Verification items for the finished model (mm, model axes). A direction names the side the tool comes from. Round coordinates to 2 decimals unless told otherwise and drop trailing zeros. Order: outer loops, then holes, each group sorted by start corner. A loop starts at its lowest first (then second) coordinate and runs counter-clockwise, first axis right, second up. Notation, with made-up numbers: M 73,-3.5 L 97,-3.5 A12 cw 97,2.5 Z; hole C 81,48 d11. An arc over 180 degrees is marked long. Return JSON: item names as keys, results as strings. Group by question number.
from build123d import *

# Parameters (mm, degrees)
SKETCH1_W           = 40
SKETCH1_H           = 20
BOSS_EXTRUDE1_DEPTH = 3
FILLET1_R           = 15


with BuildPart() as part:
    # Sketch1 → Boss-Extrude1 (new body)
    with BuildSketch(Plane.XY):
        Polygon((52, 50.85), (52, 47.85), (58, 47.85), (58, 50.85), (110, 50.85), (110, 0), (58, 0), (58, 3), (52, 3), (52, 0), (0, 0), (0, 50.85), align=None)
        with Locations((55, 25.425)):
            Rectangle(SKETCH1_W, SKETCH1_H, mode=Mode.SUBTRACT)
    extrude(amount=BOSS_EXTRUDE1_DEPTH)

    # Fillet1
    fillet1_edges = [part.edges().sort_by_distance(p)[0] for p in [
        (0, 0, 1.5),
        (110, 0, 1.5),
        (110, 50.85, 1.5),
        (0, 50.85, 1.5),
    ]]
    fillet(fillet1_edges, radius=FILLET1_R)


solid = part.part
1. Cross-section at D-D (y = 10). Enter the section's corners in (x, z), plus the area to 3 significant figures.
2. Access from +Z, -Z, +X, -X, +Y, -Y to the whole of each face (thin tool, end or side, straight path). Record for faces 4 (the face through (52, 2, 1)), 5 (the face through (52, 49, 1)), 6 (the face through (75, 25, 1)), 7 (the face through (33, 50.85, 1)).
3. Thickness scan on line 1 along Y through (x, z) = (50.5, 2.3) (3 decimals); line 2 along Y through (x, z) = (55, 0.75) (3 decimals); line 3 along X through (y, z) = (32, 2.8). Record the ranges inside material, lowest first. Write a range as from..to.
4. Go/stop test with flat-tipped pins: pin 1 (1.5 mm diameter, centred on x = 54, z = 2, fed in from -Y); pin 2 (0.9 mm diameter, centred on y = 1.5, z = 1, fed in from -X). Record where each tip stops, or that it passes through.
5. Draft check along X on faces 1 (the face through (34, 0, 1)), 2 (the face through (58, 1, 1)), 3 (the face through (4.28, 4.51, 1.52)). Enter one of: +X half, -X half, draft (parallel to the pull), parting line (faces both ways), or undercut.
6. Cross-section at C-C (y = 19). Enter the section's corners in (x, z).
7. Cross-section at B-B (z = 2.2). Enter the section's corners in (x, y) (3 decimals), plus the area to 3 significant figures.
8. Cross-section at A-A (x = 46.5). Enter the section's corners in (y, z) (3 decimals).
Computed:
{
 "1": {"outline": "M 0.86,0 L 109.14,0 L 109.14,3 L 0.86,3 Z", "area": "325 mm²"},
 "2": {"face 4": "+Z, -Z, -Y", "face 5": "+Z, -Z, +Y", "face 6": "+Z, -Z", "face 7": "+Z, -Z, +X, -X, +Y"},
 "3": {"line 1": "y = 0..15.425, 35.425..50.85", "line 2": "y = 3..15.425, 35.425..47.85", "line 3": "x = 0..35, 75..110"},
 "4": {"pin 1": "stops at y = 3", "pin 2": "stops at x = 7.6"},
 "5": {"face 1": "draft", "face 2": "undercut", "face 3": "-X half"},
 "6": {"outline": "M 0,0 L 35,0 L 35,3 L 0,3 Z; M 75,0 L 110,0 L 110,3 L 75,3 Z"},
 "7": {"outline": "M 0,15 A15 ccw 15,0 L 52,0 L 52,3 L 58,3 L 58,0 L 95,0 A15 ccw 110,15 L 110,35.85 A15 ccw 95,50.85 L 58,50.85 L 58,47.85 L 52,47.85 L 52,50.85 L 15,50.85 A15 ccw 0,35.85 Z; hole M 35,15.425 L 75,15.425 L 75,35.425 L 35,35.425 Z", "area": "4,560 mm²"},
 "8": {"outline": "M 0,0 L 15.425,0 L 15.425,3 L 0,3 Z; M 35.425,0 L 50.85,0 L 50.85,3 L 35.425,3 Z"}
}
